Autodesk Inventor part; units mm, degrees
ref_plane "Work Plane1" through (155.5635, 0, -155.5635) normal (0.7071, 0, -0.7071) x (0, 1, 0)
ref_plane "YZ Plane" through (0, 0, 0) normal (1, 0, 0) x (0, 1, 0)
ref_plane "XZ Plane" through (0, 0, 0) normal (0, 1, 0) x (-1, 0, 0)
sketch "Sketch1" plane through (0, 0, 0) normal (0, 1, 0) x (-1, 0, 0)
  arc A0 (-220, 0) -> (-67, -209.5495) centre (0, 0) ccw
  arc A1 (-217, 0) -> (-67, -206.3977) centre (0, 0) ccw
  line L0 (-220, 0) -> (-217, 0)
  line L1 (0, -220) -> (0, -217)
  line L2 (0, -220) -> (-67, -220)
  line L3 (0, -220) -> (67, -220) construction
  line L4 (-67, -220) -> (-67, -206.3977)
  line L5 (-67, -206.3977) -> (-65.0308, -207.0265)
  line L6 (-67, -206.3977) -> (-68.4601, -210.9695)
  point P0 (-67.9127, -209.2555)
  dimension "d0" = 440
  dimension "d1" = 3
  dimension "d2" = 67
  dimension "d3" = 180
  dimension "d9" = 90
extrude "Extrusion1" add sketch "Sketch1" along normal blind 92.5 contours L0 A1 L6 A0
sketch "Sketch3" plane through (0, 92.5, 0) normal (0, 1, 0) x (1, 0, 0)
  arc A0 (217, 0) -> (67, 206.3977) centre (0, 0) ccw
  arc A1 (197, 0) -> (60.8249, 187.3748) centre (0, 0) ccw
  line L0 (60.8249, 187.3748) -> (67, 206.3977)
  line L1 (197, 0) -> (217, 0)
  dimension "d10" = 20
extrude "Extrusion3" add sketch "Sketch3" against normal blind 3
sketch "Sketch4" plane through (0, 92.5, 0) normal (0, 1, 0) x (1, 0, 0)
  line L0 (197, 0) -> (220, 0)
  arc A0 (197, 0) -> (60.8249, 187.3748) centre (0, 0) ccw
  arc A1 (220, 0) -> (67.9127, 209.2555) centre (0, 0) ccw
  line L1 (196.9772, 3) -> (219.9795, 3)
  dimension "d13" = 3
extrude "Extrusion4" add sketch "Sketch4" against normal up to surface (92.5 mm away)
sketch "Sketch5" plane through (0, 89.5, 0) normal (0, -1, 0) x (1, 0, 0)
  arc A0 (60.8249, -187.3748) -> (196.9772, -3) centre (0, 0) ccw
  line L0 (60.8249, -187.3748) -> (67, -206.3977)
  arc A1 (67, -206.3977) -> (216.9793, -3) centre (0, 0) ccw
  line L1 (67, -206.3977) -> (67, -185.2566)
  line L2 (67, -206.3977) -> (88.1411, -206.3977) construction
  dimension "d16" = 90
extrude "Extrusion5" cut sketch "Sketch5" against normal through all
sketch "Sketch6" plane through (0, 0, 0) normal (0, -1, 0) x (1, 0, 0)
  line L0 (0, 0) -> (155.5635, -155.5635)
  arc A0 (67.9127, -209.2555) -> (220, 0) centre (0, 0) ccw
  line L1 (0, 0) -> (220, 0) construction
  dimension "d19" = 45
ref_plane "Work Plane1" through (155.5635, 0, -155.5635) normal (0.7071, 0, -0.7071) x (0, 1, 0)
sketch "Sketch7" plane through (155.5635, 0, -155.5635) normal (0.7071, 0, -0.7071) x (0, 1, 0)
  circle A0 centre (72.5, -12.5) radius 5
  circle A1 centre (72.5, 12.5) radius 5
  line L0 (92.5, -99.9445) -> (92.5, 155.5635)
  line L1 (0, 0) -> (103.0589, 0)
  dimension "d20" = 10
  dimension "d21" = 10
  dimension "d22" = 25
  dimension "d23" = 20
  dimension "d24" = 20
  dimension "d25" = 12.5
extrude "Extrusion6" cut sketch "Sketch7" against normal through all
properties part number "Bottom_Enclosure_2"
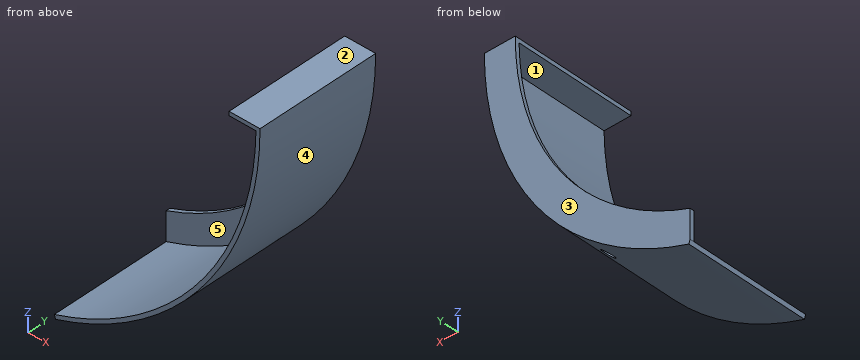
Read the model definition and answer for the solid it produces. Units are mm, in the model's axes. Face numbers are marked on the shaded views. A direction names the side the tool comes from. Round coordinates to 2 decimals unless told otherwise and drop trailing zeros. Write each loop counter-clockwise with the first axis right and the second up, starting at its lowest first coordinate (ties: lowest second). Pieces come first, ordered by that corner, then holes. Notation, with made-up numbers: M 69,0.25 L 87,0.25 A31 cw 87,39.25 Z; hole C 68,9.5 d7. An arc over 180 degrees is marked long. Use a Markdown table: item, result.
1) For a pull along Z with two mould halves and no side action, classify the marked faces 1, 2 and 3 as pulls with the +Z half, pulls with the -Z half, needs draft (parallel to the pull), parting line crosses it, or undercut.
Answers follow:
| item | result |
|---|---|
| face 1 | undercut |
| face 2 | pulls with the +Z half |
| face 3 | needs draft |
2) A tool of negligible diameter and unlimited length cuts with its end or side. For the marked faces 4 and 5, from which of +Z, -Z, +X, -X, +Y, -Y can it reach the whole face along a straight path? Write none if from no direction.
Answers follow:
| item | result |
|---|---|
| face 4 | -Z, +X, +Y, -Y |
| face 5 | -X, -Y |
3) Straight lines are drawn through the part: line 1 along Y through (x, z) = (212, -38.5); line 2 along X through (y, z) = (14.5, -77.5); line 3 along Z through (x, y) = (175, 48). For each, find the intervals that lie inside material, in ascending order. Write a range as [from, to].
Answers follow:
| item | result |
|---|---|
| line 1 | y = [89.5, 92.5] |
| line 2 | x = [202.69, 205.9] |
| line 3 | z = [-133.32, -128.31] |
4) Flat-ended cylindrical pins translate along their axes: pin 1 (4 mm diameter, centred on y = 58.5, z = -166, fed in from -X); pin 2 (5 mm diameter, centred on y = 60, z = -30, fed in from +X); pin 3 (1 mm diameter, centred on x = 94.5, y = 52, fed in from +Z). Find the tip coordinate at first contact, or state that the pin passes through.
Answers follow:
| item | result |
|---|---|
| pin 1 | stops at x = 137.35 |
| pin 2 | stops at x = 218.27 |
| pin 3 | stops at z = -195.1 |
5) The part is cut by section B-B (y = 54). Write down the section's boundary in (x, z).
Answers follow:
| item | result |
|---|---|
| outline | M 67,-206.4 L 67.91,-209.26 A220 ccw 220,0 L 197,0 A197 cw 196.98,-3 L 216.98,-3 A217 cw Z |
6) The part is cut by section A-A (x = 176). Write down the section's boundary in (y, z), plus the area to 3 significant figures.
Answers follow:
| item | result |
|---|---|
| outline | M 0,-132 L 92.5,-132 L 92.5,-88.5 L 89.5,-88.5 L 89.5,-126.94 L 0,-126.94 Z |
| area | 584 mm2 |
